Verification items for the finished model (mm, model axes). Give positions to 0.01 mm unless a question says otherwise; leave off trailing zeros. Order: outer loops, then holes, each group sorted by start corner. A loop starts at its lowest first (then second) coordinate and runs counter-clockwise, first axis right, second up. Notation, with made-up numbers: (-24, 18.25) -> (-18, 18.25) arc R29 cw to (-18, 39.25) -> close; hole circle Ø11 at (75, -37). An arc over 180 degrees is marked (long way). One line per question, with ' | ' between items. Start each with the question number.
Q1. Material ranges on probe 1 along Z at (x, y) = (-8, 0.5); probe 2 along Y at (x, z) = (-12.7, 111.75); probe 3 along Z at (x, y) = (49, 3), recorded low to high. Write a range as [from, to].
Q2. Go/stop test with flat-tipped pins: pin 1 (1 mm diameter, centred on y = 5, z = 79.5, fed in from -X); pin 2 (3 mm diameter, centred on x = -12.7, y = 3.175, fed in from +Z); pin 3 (3 mm diameter, centred on x = -38, y = 2.5, fed in from +Z). Record where each tip stops, or that it passes through.
Q3. Section check A-A on z = -8. Record the cut outline in (x, y).
Q4. Section check B-B on z = 40.5. Record the cut outline in (x, y).
from build123d import *

# Parameters (mm, degrees)
SKETCH2_W                       = 128
SKETCH2_H                       = 127
BOSS_EXTRUDE1_DEPTH             = 6.35
BOSS_EXTRUDE2_DEPTH             = 6.35
F_6_32_TAPPED_HOLE1_D           = 2.7051
F_6_32_TAPPED_HOLE1_DEPTH       = 9.398
F_6_32_TAPPED_HOLE1_CBORE_D     = 3.5052
F_6_32_TAPPED_HOLE1_CBORE_DEPTH = 7.112
F_6_32_TAPPED_HOLE1_TIP         = 0.81269403


with BuildPart() as part:
    # Sketch2 → Boss-Extrude1 (new body)
    with BuildSketch(Plane(origin=(0, 0, 0), x_dir=(1, 0, 0), z_dir=(0, 1, 0))):
        Rectangle(SKETCH2_W, SKETCH2_H)
        with BuildLine():
            Line((29.695725746, 58.5), (-29.695725746, 58.5))
            ThreePointArc((-29.695725746, 58.5), (-46.315550876, 45.606106313), (-59, 28.825884855))
            Line((-59, 28.825884855), (-59, -28.825884855))
            ThreePointArc((-59, -28.825884855), (-46.315550876, -45.606106313), (-29.695725746, -58.5))
            Line((-29.695725746, -58.5), (29.695725746, -58.5))
            ThreePointArc((29.695725746, -58.5), (46.315550876, -45.606106313), (59, -28.825884855))
            Line((59, -28.825884855), (59, 28.825884855))
            ThreePointArc((59, 28.825884855), (46.315550876, 45.606106313), (29.695725746, 58.5))
        make_face(mode=Mode.SUBTRACT)
    extrude(amount=BOSS_EXTRUDE1_DEPTH)

    # Sketch3 → Boss-Extrude2 (add)
    with BuildSketch(Plane(origin=(0, 6.35, 0), x_dir=(1, 0, 0), z_dir=(0, 1, 0))):
        Polygon((-64, -63.5), (-19.05, -114.3), (19.05, -114.3), (64, -63.5), align=None)
        Polygon((-49.902284759, -69.85), (-16.189784759, -107.95), (16.189784759, -107.95), (49.902284759, -69.85), align=None, mode=Mode.SUBTRACT)
    extrude(amount=-BOSS_EXTRUDE2_DEPTH)

    # #6-32 Tapped Hole1
    with Locations(Plane.XY.offset(114.3)):
        with Locations((-12.7, 3.175), (12.7, 3.175)):
            CounterBoreHole(F_6_32_TAPPED_HOLE1_D / 2, F_6_32_TAPPED_HOLE1_CBORE_D / 2, F_6_32_TAPPED_HOLE1_CBORE_DEPTH, depth=F_6_32_TAPPED_HOLE1_DEPTH)
            with Locations((0, 0, -(F_6_32_TAPPED_HOLE1_DEPTH + F_6_32_TAPPED_HOLE1_TIP / 2))):  # 118° drill point
                Cone(0, F_6_32_TAPPED_HOLE1_D / 2, F_6_32_TAPPED_HOLE1_TIP, mode=Mode.SUBTRACT)


solid = part.part
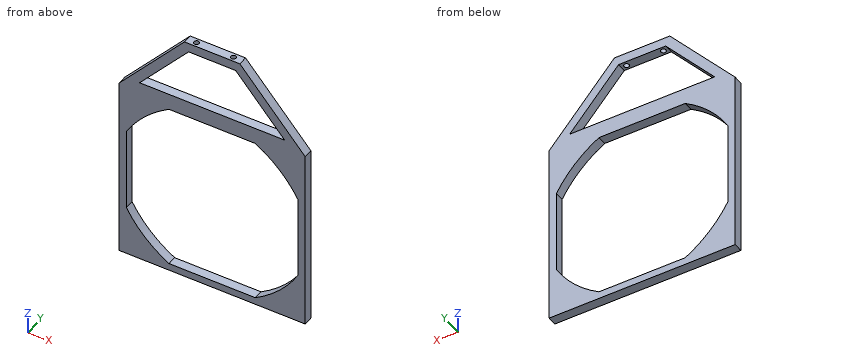
Filled in:
1) probe 1: [-63.5, -58.5], [58.5, 69.85], [107.95, 114.3] | probe 2: [0, 1.42], [4.93, 6.35] | probe 3: [-63.5, -42.75], [42.75, 69.85], [70.87, 80.45]
2) pin 1: x = -50.28 | pin 2: z = 69.85 | pin 3: z = 94.58
3) outline: (-64, 0) -> (-59, 0) -> (-59, 6.35) -> (-64, 6.35) -> close; (59, 0) -> (64, 0) -> (64, 6.35) -> (59, 6.35) -> close
4) outline: (-64, 0) -> (-50.94, 0) -> (-50.94, 6.35) -> (-64, 6.35) -> close; (50.94, 0) -> (64, 0) -> (64, 6.35) -> (50.94, 6.35) -> close
